```python
from build123d import *

# Parameters (mm, degrees)
CROQUIS2_R = 2.5


with BuildPart() as part:
    # Barrer1: sweep along a path in Croquis1
    with BuildLine(Plane(origin=(0, 0, 0), x_dir=(1, 0, 0), z_dir=(0, 1, 0))) as barrer1_path:
        Line((-200.934, 131.5), (200.934, 131.5))
        Line((200.934, 131.5), (200.934, -131.5))
        Line((200.934, -131.5), (-200.934, -131.5))
        Line((-200.934, -131.5), (-200.934, 131.5))
    # Croquis2 → Barrer1 (sweep)
    with BuildSketch(Plane(origin=(0, 0, 0), x_dir=(0, 0, -1), z_dir=(1, 0, 0))):
        Polygon((-134.849716447, 9.750635048), (-134.849716447, 9.390635048), (-134.344716447, 9.390635048), (-134.344716447, 8.020635048), (-136.679716447, 8.020635048), (-136.679716447, 6.720635048), (-135.123236313, 5.163216334), (-127.876765738, 5.163216334), (-126.320285605, 6.720635048), (-126.320285605, 8.020635048), (-128.655285605, 8.020635048), (-128.655285605, 9.390635048), (-128.150285605, 9.390635048), (-128.150285605, 9.750635048), (-121.749166204, 9.750635048), (-121.749166204, 3.185392978), (-122.109166138, 3.185175958), (-122.108861707, 2.680176049), (-123.478861458, 2.679350168), (-123.480269074, 5.014349744), (-124.780268838, 5.01356606), (-126.336748971, 3.456147346), (-126.336748971, -3.456060512), (-124.780268838, -5.013479227), (-123.480269074, -5.01426291), (-123.478861458, -2.679263334), (-122.108861707, -2.680089216), (-122.109166138, -3.185089124), (-121.749166204, -3.185306144), (-121.749166204, -9.750548215), (-128.150285605, -9.750548215), (-128.150285605, -9.390548215), (-128.655285605, -9.390548215), (-128.655285605, -8.020548215), (-126.320285605, -8.020548215), (-126.320285605, -6.720548215), (-127.876765738, -5.1631295), (-135.123236313, -5.1631295), (-136.679716447, -6.720548215), (-136.679716447, -8.020548215), (-134.344716447, -8.020548215), (-134.344716447, -9.390548215), (-134.849716447, -9.390548215), (-134.849716447, -9.750548215), (-141.250835848, -9.750548215), (-141.250835848, -3.185306144), (-140.890835913, -3.185089124), (-140.891140344, -2.680089216), (-139.521140593, -2.679263334), (-139.519732977, -5.01426291), (-138.219733214, -5.013479227), (-136.66325308, -3.456060512), (-136.66325308, 3.456147346), (-138.219733214, 5.01356606), (-139.519732977, 5.014349744), (-139.521140593, 2.679350168), (-140.891140344, 2.680176049), (-140.890835913, 3.185175958), (-141.250835848, 3.185392978), (-141.250835848, 9.750635048), align=None)
        with Locations((-131.500001026, 4.3417e-05)):
            Circle(CROQUIS2_R, mode=Mode.SUBTRACT)
    sweep(path=barrer1_path.line, transition=Transition.RIGHT)


solid = part.part
```
Could you check a few things on this model? Use its own coordinates, in mm. Round coordinates to 2 decimals unless told otherwise and drop trailing zeros. One line per question, with ' | ' between items. Start each with the question number.
(1) Suppose I cut it at A-A on z = -28.5. Count the separate pieces of the cut face and the enclosed holes in it, then the cut area to 3 significant figures.
(2) Thinking about a two-plate mould opening in X: for faces 1 (the face through (62, 5.163, 131)), 2 (the face through (1, 9.751, 137)), 3 (the face through (62, -5.163, 129)), which applies, +X half, -X half, draft (parallel to the pull), parting line (faces both ways), or undercut?
(3) For P1, Ø4, axis at x = 200.93, y = 0, coming from the -Z side; P2, Ø6, axis at x = 136.5, y = 3, coming from the +Z side; P3, Ø12, axis at x = 101.5, z = 112, coming from the -Y side; P4, Ø2, axis at x = -143, y = 1.5, coming from the +Z side, each with a flat end and sliding along its axis, tell me the tip position at first contact or that it passes through.
(4) Please list where these lines run through material, in increasing order: line 1 along X through (y, z) = (-7, 100.5); line 2 along X through (y, z) = (-3, -6); line 3 along Z through (x, y) = (35, -3.5).
Geometry results:
1) separate pieces: 2 | enclosed holes: 2 | area: 428 mm²
2) face 1: undercut | face 2: draft | face 3: undercut
3) P1: z = -136.66 | P2: z = 141.25 | P3: through | P4: z = 136.66
4) line 1: -210.68 to -206.11, -195.75 to -191.18, 191.18 to 195.75, 206.11 to 210.68 | line 2: -210.32 to -208.95, -206.1 to -195.77, -192.91 to -191.54, 191.54 to 192.91, 195.77 to 206.1, 208.95 to 210.32 | line 3: -141.25 to -139.52, -136.71 to -126.29, -123.48 to -121.75, 121.75 to 123.48, 126.29 to 136.71, 139.52 to 141.25
